Read the model definition and answer for the solid it produces. Units are mm, in the model's axes. A direction names the side the tool comes from. Give positions to 0.01 mm unless a question says otherwise; leave off trailing zeros. Loops run counter-clockwise (first coordinate to the right, second up) from the corner with the lowest first, then second, coordinate; pieces in that order, holes last. Notation, with made-up numbers: (2.25, 21) -> (59.25, 21) arc R10 ccw to (59.25, 38) -> close; hole circle Ø9 at (37.5, -6.75). An arc over 180 degrees is marked (long way). Write each question's results on one line, items separated by ' | '. Start each with the question number.
Item 1: Which of the six approach directions +Z, -Z, +X, -X, +Y, -Y give full straight-line access (tool end or side, diameter ignored) to faces 1 (the flat face through (3, 23.812, -3)), 2 (the flat face through (3, 1.588, -73)), 3 (the flat face through (3, 13, -66.675))?
Item 2: Find the intervals of material crossed by line 1 (Y direction, x = 4, z = -73); line 2 (Y direction, x = 5, z = -40) (3 decimals); line 3 (Y direction, x = 1.5, z = -47) (3 decimals), in increasing order.
Item 3: Section A-A on z = -48.5 is taken. Write down the section's boundary in (x, y) (3 decimals).
Item 4: Section B-B on x = 4.5 is taken. State how many separate pieces and enclosed holes the cut face has, and give its area (3 significant figures).
Item 5: Each of these flat-tipped pins is pushed along its axis until it touches: P1, Ø2.5, axis at y = 7.94, z = -3.18, coming from the +X side; P2, Ø0.5, axis at x = 2.5, y = 1, coming from the +Z side; P3, Ø1.9, axis at x = 4, z = -73, coming from the -Y side; P4, Ø1.9, axis at x = 2, z = -73, coming from the +Y side. Where does it stop, or does it pass through?
Item 6: Determine the mould class of faces 4 (the flat face through (3, 1, -69.85)), 5 (the flat face through (0, 13, -38)), 6 (the flat face through (3, 13, -9.525)), 7 (the flat face through (3, 1, -6.35)) for opening direction Z: +Z half, -Z half, draft (parallel to the pull), parting line (faces both ways), or undercut.
```python
from build123d import *

# Parameters (mm, degrees)
BOSS_EXTRUDE1_DEPTH                               = 6.35
CSK_FOR_6_FLAT_HEAD_MACHINE_SCREW_100_D           = 3.7973
CSK_FOR_6_FLAT_HEAD_MACHINE_SCREW_100_CSINK_D     = 7.0866
CSK_FOR_6_FLAT_HEAD_MACHINE_SCREW_100_CSINK_ANGLE = 100
CUT_EXTRUDE1_DEPTH                                = 81.572467382


with BuildPart() as part:
    # Sketch1 → Boss-Extrude1 (new body)
    with BuildSketch(Plane(origin=(0, 0, 0), x_dir=(0, 0, -1), z_dir=(1, 0, 0))):
        Polygon((69.85, 25.4), (38.1, 25.4), (38.1, 0), (69.85, 0), (69.85, 1.5875), (76.2, 1.5875), (76.2, 23.8125), (69.85, 23.8125), align=None)
        Polygon((38.1, 0), (38.1, 25.4), (6.35, 25.4), (6.35, 23.8125), (0, 23.8125), (0, 1.5875), (6.35, 1.5875), (6.35, 0), align=None)
    extrude(amount=BOSS_EXTRUDE1_DEPTH)

    # CSK for #6 Flat Head Machine Screw (100)1 (through all)
    with Locations(Plane.ZY):
        with Locations((-73.025, 17.4625), (-73.025, 7.9375), (-3.175, 17.4625), (-3.175, 7.9375)):
            CounterSinkHole(CSK_FOR_6_FLAT_HEAD_MACHINE_SCREW_100_D / 2, CSK_FOR_6_FLAT_HEAD_MACHINE_SCREW_100_CSINK_D / 2, counter_sink_angle=CSK_FOR_6_FLAT_HEAD_MACHINE_SCREW_100_CSINK_ANGLE)

    # Sketch4 → Cut-Extrude1 (cut, through all)
    with BuildSketch(Plane.ZY):
        Polygon((-42.116092628, 12.7), (-66.675, 20.886302457), (-66.675, 4.513697543), align=None)
        Polygon((-13.541092628, 22.225), (-62.658907372, 22.225), (-38.1, 14.038697543), align=None)
        Polygon((-9.525, 20.886302457), (-34.083907372, 12.7), (-9.525, 4.513697543), align=None)
        Polygon((-13.541092628, 3.175), (-38.1, 11.361302457), (-62.658907372, 3.175), align=None)
    extrude(amount=-CUT_EXTRUDE1_DEPTH, mode=Mode.SUBTRACT)


solid = part.part
```
Findings:
1) face 1: +Z, +X, -X, +Y | face 2: -Z, +X, -X, -Y | face 3: +X, -X
2) line 1: 1.59 to 6.04, 9.84 to 15.56, 19.36 to 23.81 | line 2: 0 to 3.175, 10.728 to 14.672, 22.225 to 25.4 | line 3: 0 to 3.175, 8.395 to 11.072, 14.328 to 17.005, 22.225 to 25.4
3) outline: (0, 0) -> (6.35, 0) -> (6.35, 3.175) -> (0, 3.175) -> close; (0, 7.895) -> (6.35, 7.895) -> (6.35, 10.572) -> (0, 10.572) -> close; (0, 14.828) -> (6.35, 14.828) -> (6.35, 17.505) -> (0, 17.505) -> close; (0, 22.225) -> (6.35, 22.225) -> (6.35, 25.4) -> (0, 25.4) -> close
4) separate pieces: 1 | enclosed holes: 8 | area: 1,050 mm2
5) P1: through | P2: z = -6.35 | P3: y = 1.59 | P4: y = 23.81
6) face 4: -Z half | face 5: draft | face 6: undercut | face 7: +Z half
